Autodesk Inventor part; units mm, degrees
ref_plane "YZ Plane" through (0, 0, 0) normal (1, 0, 0) x (0, 1, 0)
ref_plane "XZ Plane" through (0, 0, 0) normal (0, 1, 0) x (-1, 0, 0)
ref_plane "XY Plane" through (0, 0, 0) normal (0, 0, 1) x (1, 0, 0)
sketch "Эскиз1" plane through (0, 0, 0) normal (0, 1, 0) x (-1, 0, 0)
  line L0 (0, 0) -> (-200, 0)
  line L1 (-200, 0) -> (-200, -30)
  line L2 (-200, -30) -> (0, -30)
  line L3 (0, -30) -> (0, 0)
  dimension "d0" = 200
  dimension "d1" = 30
extrude "Выдавливание1" add sketch "Эскиз1" along normal blind 80
chamfer "Фаска1" distance 30 angle 45 2 edges at (0, 40, 0) (200, 40, 0)
properties part number "dou_short_round" material "Красное дерево"
For this review, take the finished solid that the model builds, in its own axes (mm). Coordinates: 2 decimals unless noted, no trailing zeros. Write each loop counter-clockwise with the first axis right and the second up, starting at its lowest first coordinate (ties: lowest second). Pieces come first, ordered by that corner, then holes. Notation, with made-up numbers: (21, 5.5) -> (64, 5.5) arc R34 ccw to (64, 36.5) -> close; hole circle Ø4 at (69.5, 75). An arc over 180 degrees is marked (long way). Put each result on its own line as item: value.
Q1. Take a section at B-B, the plane z = -7. State the section outline as (x, y) points, then the cut area to 3 significant figures.
From the geometry:
outline: (23, 0) -> (177, 0) -> (177, 80) -> (23, 80) -> close
area: 12,300 mm2
Q2. Take a section at C-C, the plane x = 176.5. State the section outline as (y, z) points, then the cut area to 3 significant figures.
From the geometry:
outline: (0, -30) -> (80, -30) -> (80, -6.5) -> (0, -6.5) -> close
area: 1,880 mm2
Q3. Clearance check with a flat-ended pin moving along its axis: pin 1 Ø1.5 at (y, z) = (55, -6) entering from -X. State where the tip first meets the part, or that it passes through.
From the geometry:
pin 1: stops at x = 23.25
Q4. Wall thickness on L1, parallel to Z at x = 8.5, y = 4; L2, parallel to X at y = 43.5, z = -11.75; L3, parallel to X at y = 50, z = -13.25: over which ranges is each line inside the solid? List them lowest first.
From the geometry:
L1: z = -30 to -21.5
L2: x = 18.25 to 181.75
L3: x = 16.75 to 183.25
Q5. The part is to be moulded in two halves that separate along Z. For faces 1 (the flat face through (101, 39, -30)), 2 (the flat face through (101, 0, -15)), 3 (the flat face through (99, 39, 0)), say which applies: +Z half, -Z half, draft (parallel to the pull), parting line (faces both ways), or undercut.
From the geometry:
face 1: -Z half
face 2: draft
face 3: +Z half
